Input: part model. Units: mm. Frame: model coordinates. Face numbers are marked on the shaded views. Coordinates: 2 decimals unless noted, no trailing zeros. Write each loop counter-clockwise with the first axis right and the second up, starting at its lowest first coordinate (ties: lowest second). Pieces come first, ordered by that corner, then holes. Notation, with made-up numbers: (9.25, 89) - (48.25, 89) arc R8 cw to (48.25, 99) - close; hole circle Ø7 at (72, 57). An arc over 180 degrees is marked (long way). Put each result on its own line as item: value. Start each with the question number.
1. Pull-direction query (X, two-part tool) for the marked faces 1, 2, 3 and 4; classes: released by +X, released by -X, zero draft, split by the parting line, or undercut.
2. Cut plane B-B, the plane y = -40. Return loops of the section in (x, z), and give its area (3 significant figures).
3. Line query: line 1 (Y direction, x = 0, z = -10.4); line 2 (X direction, y = -55, z = -6.25); line 3 (X direction, y = -58.5, z = -5.5). Output: solid intervals per line, ascending.
4. Cut plane C-C, the plane x = -3.5. Return loops of the section in (y, z), and give its area (4 significant figures).
5. Cut plane A-A, the plane x = 0. Return loops of the section in (y, z), and give its area (3 significant figures).
6. Pin query (flat end, axial travel): pin 1 (5 mm diameter, centred on x = -3, y = -44, fed in from +Z); pin 2 (3 mm diameter, centred on x = 0, y = -70, fed in from -Z). Return the tip coordinate at first contact, or that it passes through.
from build123d import *

# Parameters (mm, degrees)
PAD003_DEPTH    = 25
SKETCH030_R     = 1.25
POCKET005_DEPTH = 12.001
CHAMFER007_SIZE = 0.3
CHAMFER008_SIZE = 0.5


with BuildPart() as part:
    # Sketch028 → Pad003 (new body, symmetric)
    with BuildSketch(Plane.XZ):
        with BuildLine():
            Line((-7.5, -5), (-7.5, -6.5))
            ThreePointArc((-7.5, -6.5), (-7.353553, -6.853553), (-7, -7))
            Line((-7, -7), (7, -7))
            ThreePointArc((7, -7), (7.353553, -6.853553), (7.5, -6.5))
            Line((7.5, -6.5), (7.5, -5))
            Line((7.5, -5), (12, -5))
            Line((12, -5), (13, -6))
            Line((13, -6), (13, -11))
            Line((13, -11), (12, -12))
            Line((12, -12), (-12, -12))
            Line((-13, -11), (-12, -12))
            Line((-13, -11), (-13, -6))
            Line((-13, -6), (-12, -5))
            Line((-12, -5), (-7.5, -5))
        make_face()
    extrude(amount=PAD003_DEPTH, both=True)

    # Sketch030 → Pocket005 (cut, through all)
    with BuildSketch(Plane.XY):
        with Locations((0, 15)):
            Circle(SKETCH030_R)
        with Locations((0, -15)):
            Circle(SKETCH030_R)
    extrude(amount=-POCKET005_DEPTH, mode=Mode.SUBTRACT)

    # Chamfer007
    chamfer007_edges = [part.edges().sort_by_distance(p)[0] for p in [
        (-7.5, 0, -5),
        (7.5, 0, -5),
        (-1.25, 15, -7),
        (-1.25, -15, -7),
        (-1.25, 15, -12),
        (-1.25, -15, -12),
    ]]
    chamfer(chamfer007_edges, length=CHAMFER007_SIZE)

    # Chamfer008
    chamfer008_edges = [part.edges().sort_by_distance(p)[0] for p in [
        (-9.9, -25, -5),
        (-7.65, -25, -5.15),
        (-12.5, -25, -5.5),
        (-7.5, -25, -5.9),
        (-13, -25, -8.5),
        (-7.353553, -25, -6.853553),
        (-12.5, -25, -11.5),
        (0, -25, -7),
        (0, -25, -12),
        (7.353553, -25, -6.853553),
        (12.5, -25, -11.5),
        (7.5, -25, -5.9),
        (13, -25, -8.5),
        (7.65, -25, -5.15),
        (12.5, -25, -5.5),
        (9.9, -25, -5),
        (-9.9, 25, -5),
        (-7.65, 25, -5.15),
        (-12.5, 25, -5.5),
        (-7.5, 25, -5.9),
        (-13, 25, -8.5),
        (-7.353553, 25, -6.853553),
        (-12.5, 25, -11.5),
        (0, 25, -7),
        (0, 25, -12),
        (7.353553, 25, -6.853553),
        (12.5, 25, -11.5),
        (7.5, 25, -5.9),
        (13, 25, -8.5),
        (7.65, 25, -5.15),
        (12.5, 25, -5.5),
        (9.9, 25, -5),
    ]]
    chamfer(chamfer008_edges, length=CHAMFER008_SIZE)


with BuildPart() as part_1:
    # Body004 placement: moved
    add(part.part.moved(Location((0, -55, 0))))


solid = part_1.part
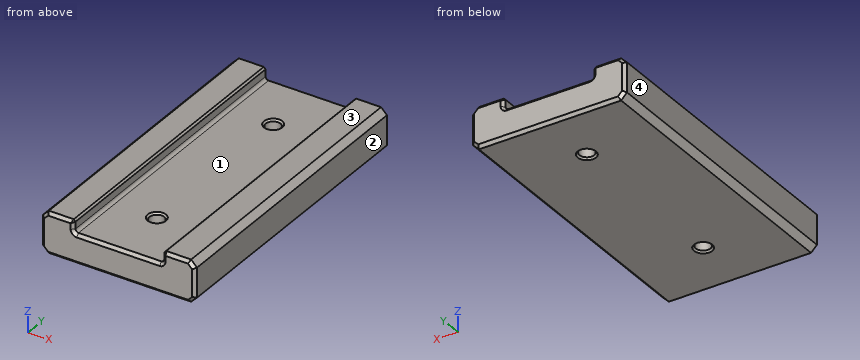
Report:
1. face 1: undercut
1. face 2: released by +X
1. face 3: zero draft
1. face 4: released by -X
2. outline: (-13, -11) - (-12, -12) - (-1.55, -12) - (-1.25, -11.7) - (-1.25, -7.3) - (-1.55, -7) - (-7, -7) arc R0.5 cw to (-7.5, -6.5) - (-7.5, -5.3) - (-7.8, -5) - (-12, -5) - (-13, -6) - close; (1.25, -11.7) - (1.55, -12) - (12, -12) - (13, -11) - (13, -6) - (12, -5) - (7.8, -5) - (7.5, -5.3) - (7.5, -6.5) arc R0.5 cw to (7, -7) - (1.55, -7) - (1.25, -7.3) - close
2. area: 137 mm^2
3. line 1: y = -80 to -71.25, -68.75 to -41.25, -38.75 to -30
3. line 2: x = -13 to -7.5, 7.5 to 13
3. line 3: x = -12.5 to -7.5, 7.5 to 12.5
4. outline: (-80, -11.5) - (-79.5, -12) - (-30.5, -12) - (-30, -11.5) - (-30, -7.5) - (-30.5, -7) - (-79.5, -7) - (-80, -7.5) - close
4. area: 249.5 mm^2
5. outline: (-80, -11.5) - (-79.5, -12) - (-71.55, -12) - (-71.25, -11.7) - (-71.25, -7.3) - (-71.55, -7) - (-79.5, -7) - (-80, -7.5) - close; (-68.75, -11.7) - (-68.45, -12) - (-41.55, -12) - (-41.25, -11.7) - (-41.25, -7.3) - (-41.55, -7) - (-68.45, -7) - (-68.75, -7.3) - close; (-38.75, -11.7) - (-38.45, -12) - (-30.5, -12) - (-30, -11.5) - (-30, -7.5) - (-30.5, -7) - (-38.45, -7) - (-38.75, -7.3) - close
5. area: 224 mm^2
6. pin 1: stops at z = -7
6. pin 2: stops at z = -11.95
